Build history of the part. All positions in model axes, mm. A direction names the side the tool comes from. Round coordinates to 2 decimals unless told otherwise and drop trailing zeros. Write each loop counter-clockwise with the first axis right and the second up, starting at its lowest first coordinate (ties: lowest second). Pieces come first, ordered by that corner, then holes. Notation, with made-up numbers: (80, -33.5) - (93, -33.5) arc R29 ccw to (93, -9.5) - close; hole circle Ø9 at (-0.75, 2). An arc over 180 degrees is marked (long way). Answer as a JSON object with one key per item and string values. Group by question number.
Item 1: Probe line 1 (Y direction, x = 0, z = 4.5); line 2 (Z direction, x = -1, y = 3); line 3 (Y direction, x = -1, z = -4.25). List the from-to ranges inside material, lowest first. Write a range as from..to.
Item 2: Flat gauge pins, fed straight in: pin 1 (0.9 mm diameter, centred on y = 0.5, z = -5, fed in from +X); pin 2 (0.7 mm diameter, centred on y = 1.5, z = -1, fed in from -X). Where does each tip first touch, or does it go through?
Item 3: Which spindle directions (+Z, -Z, +X, -X, +Y, -Y) get a long thin tool onto all of the face, cutting with end or side? Do faces 1 (the flat face through (0, 3, 0)), 2 (the cylindrical face through (2.5, 0.1, 3.5)), 3 (the cylindrical face through (0, 2, -5)). Say none if no direction does.
Item 4: Slice it at A-A, the plane x = 0. List the corners of the cut face in (y, z).
Item 5: Slice it at B-B, the plane y = 0. List the corners of the cut face in (x, z), then the cut area to 3 significant figures.
Item 6: Two-plate mould, pull along Y, no slides. Class faces 4 (the cylindrical face through (3.34, 1.05, -0.1)), 5 (the flat face through (-1.5, 0, 1)), 6 (the flat face through (0, -3, 0)): +Y half, -Y half, draft (parallel to the pull), parting line (faces both ways), or undercut.
Item 7: Slice it at D-D, the plane x = 1. Give the number of separate pieces and of enclosed holes in the cut face, then the cut area to 3 significant figures.
Item 8: Slice it at C-C, the plane z = 5.75. List the corners of the cut face in (x, y).
from build123d import *
from build123d.topology import SkipClean

# Parameters (mm, degrees)
EXTRUDE_1_DEPTH                 = 7.5
EXTRUDE_1_DEPTH_BACK            = 7.5
SKETCH_1_R                      = 3.5
CUT_EXTRUDE_1_REACH             = 10.986
CUT_EXTRUDE_1_DIRECTION_2_REACH = 10.986
FILLET_1_R                      = 0.2
SKETCH_3_R                      = 2.5
CUT_EXTRUDE_2_DEPTH             = 0.5
CUT_EXTRUDE_3_DEPTH             = 7
CHAMFER_1_SIZE                  = 0.5
CHAMFER_2_SIZE                  = 0.5


with BuildPart() as part:
    # 草图1 → 凸台-拉伸1 (new, two sides: drawn at the far end of the back side and taken through both)
    with BuildSketch(Plane.XY.offset(-EXTRUDE_1_DEPTH_BACK)):
        Circle(SKETCH_1_R)
        with BuildLine():
            Line((-1.25, 1.5612495), (-1.25, -1.5612495))
            ThreePointArc((-1.25, -1.5612495), (0, -2), (1.25, -1.5612495))
            Line((1.25, -1.5612495), (1.25, 1.5612495))
            ThreePointArc((1.25, 1.5612495), (0, 2), (-1.25, 1.5612495))
        make_face(mode=Mode.SUBTRACT)
    extrude(amount=EXTRUDE_1_DEPTH + EXTRUDE_1_DEPTH_BACK)

    # 草图2 → 切除-拉伸1 (cut, up to next)
    with BuildSketch(Plane(origin=(0, 0, 0), x_dir=(1, 0, 0), z_dir=(0, 1, 0)), mode=Mode.PRIVATE) as cut_extrude_1_sk1:
        Polygon((0, 0), (-1.5, 0), (-1.5, 2.25), (1.5, 2.25), (1.5, 0), align=None)
    cut_extrude_1_tool1 = extrude(cut_extrude_1_sk1.sketch, amount=-CUT_EXTRUDE_1_REACH, mode=Mode.PRIVATE) & part.part
    add(cut_extrude_1_tool1.solids().sort_by_distance((0, 0, -1.125))[0], mode=Mode.SUBTRACT)

    # 草图2 → 切除-拉伸1 direction 2 (cut, up to next)
    with BuildSketch(Plane(origin=(0, 0, 0), x_dir=(1, 0, 0), z_dir=(0, 1, 0)), mode=Mode.PRIVATE) as cut_extrude_1_direction_2_sk1:
        Polygon((0, 0), (-1.5, 0), (-1.5, 2.25), (1.5, 2.25), (1.5, 0), align=None)
    cut_extrude_1_direction_2_tool1 = extrude(cut_extrude_1_direction_2_sk1.sketch, amount=CUT_EXTRUDE_1_DIRECTION_2_REACH, mode=Mode.PRIVATE) & part.part
    add(cut_extrude_1_direction_2_tool1.solids().sort_by_distance((0, 0, -1.125))[0], mode=Mode.SUBTRACT)

    # 圆角1
    fillet_1_edges = [part.edges().sort_by_distance(p)[0] for p in [
        (-3.5, 0, -7.5),
        (-3.5, 0, 7.5),
    ]]
    fillet(fillet_1_edges, radius=FILLET_1_R)

    # 草图3 → 切除-拉伸2 (cut)
    with BuildSketch(Plane.XY.offset(7.5)):
        Circle(SKETCH_3_R)
    extrude(amount=-CUT_EXTRUDE_2_DEPTH, mode=Mode.SUBTRACT)

    # 草图4 → 切除-拉伸3 (cut)
    with SkipClean():  # the faces are left unmerged after this step: merging them gives an invalid solid
        with BuildSketch(Plane.XY.offset(7)):
            with BuildLine():
                Line((-1.5, 0), (-1.5, 2))
                ThreePointArc((-1.5, 2), (2.5, 0), (-1.5, -2))
                Line((-1.5, -2), (-1.5, 0))
            make_face()
        extrude(amount=-CUT_EXTRUDE_3_DEPTH, mode=Mode.SUBTRACT)

    # 倒角1
    # the kernel refuses this chamfer: 0.5 mm, written as the material it takes off along each edge
    with BuildSketch(Plane(origin=(0, 0, 7.5), x_dir=(1, 0, 0), z_dir=(0, -1, 0))) as chamfer_1_piece_1_section:
        Polygon((2.5 + CHAMFER_1_SIZE, 0), (2.5, -CHAMFER_1_SIZE), (2.5, 0), align=None)
    chamfer_1_piece_1 = revolve(axis=Axis((0, 0, 7.5), (0, 0, 1)), mode=Mode.PRIVATE)
    chamfer_1_piece_1 = split(chamfer_1_piece_1, bisect_by=Plane(origin=(-1.5, 2.458621217, 7.265320049), z_dir=(1, 0, 0)), keep=Keep.TOP, mode=Mode.PRIVATE)
    chamfer_1_piece_1 = split(chamfer_1_piece_1, bisect_by=Plane(origin=(1.229310608, 2.458621217, 7), z_dir=(0, 0, 1)), keep=Keep.TOP, mode=Mode.PRIVATE)
    add(chamfer_1_piece_1, mode=Mode.SUBTRACT)
    with BuildSketch(Plane(origin=(0, 0, 7.5), x_dir=(1, 0, 0), z_dir=(0, -1, 0))) as chamfer_1_piece_2_section:
        Polygon((2.5 + CHAMFER_1_SIZE, 0), (2.5, -CHAMFER_1_SIZE), (2.5, 0), align=None)
    chamfer_1_piece_2 = revolve(axis=Axis((0, 0, 7.5), (0, 0, 1)), mode=Mode.PRIVATE)
    chamfer_1_piece_2 = split(chamfer_1_piece_2, bisect_by=Plane(origin=(-1.5, 0, 7.263385129), z_dir=(-1, 0, 0)), keep=Keep.TOP, mode=Mode.PRIVATE)
    chamfer_1_piece_2 = split(chamfer_1_piece_2, bisect_by=Plane(origin=(-2.750757007, 0, 7), z_dir=(0, 0, 1)), keep=Keep.TOP, mode=Mode.PRIVATE)
    add(chamfer_1_piece_2, mode=Mode.SUBTRACT)
    with BuildSketch(Plane(origin=(-1.5, -3.285841494, 7), x_dir=(0.02749587661058651, 0, -0.9996219169112968), z_dir=(0, 1, 0))) as chamfer_1_piece_3_section:
        Polygon((CHAMFER_1_SIZE * 0.999621916911, CHAMFER_1_SIZE * 0.0274958766106), (-CHAMFER_1_SIZE * 0.0274958766106, CHAMFER_1_SIZE * 0.999621916911), (0, 0), align=None)
    chamfer_1_piece_3 = extrude(amount=6.571682988, mode=Mode.PRIVATE)
    chamfer_1_piece_3 = chamfer_1_piece_3 & Plane(origin=(0, 0, 6.830829646), x_dir=(-0.5999999999999999, 0.8, 0), z_dir=(0, 0, 1)) * Cylinder(2.5, 16, mode=Mode.PRIVATE)
    add(chamfer_1_piece_3, mode=Mode.SUBTRACT)

    # 倒角2
    chamfer_2_edges = [part.edges().sort_by_distance(p)[0] for p in [
        (-1.25, 0, -7.5),
        (0, -2, -7.5),
        (1.25, 0, -7.5),
        (0, 2, -7.5),
    ]]
    chamfer(chamfer_2_edges, length=CHAMFER_2_SIZE)


solid = part.part
Geometry says:
{
 "1": {"line 1": "y = -3.5..-2.5, 2.5..3.5", "line 2": "z = -7.5..-2.25, 0..7.5", "line 3": "y = -3.35..-1.73, 1.73..3.35"},
 "2": {"pin 1": "stops at x = 3.5", "pin 2": "stops at x = -3.31"},
 "3": {"face 1": "+Y, -Y", "face 2": "+Z", "face 3": "+Z, -Z"},
 "4": {"outline": "(-3.5, -7.3) arc R0.2 ccw to (-3.3, -7.5) - (-2.5, -7.5) - (-2, -7) - (-2, -2.25) - (-3.5, -2.25) - close; (-3.5, 0) - (-2.5, 0) - (-2.5, 7) - (-3, 7.5) - (-3.3, 7.5) arc R0.2 ccw to (-3.5, 7.3) - close; (2, -7) - (2.5, -7.5) - (3.3, -7.5) arc R0.2 ccw to (3.5, -7.3) - (3.5, -2.25) - (2, -2.25) - close; (2.5, 0) - (3.5, 0) - (3.5, 7.3) arc R0.2 ccw to (3.3, 7.5) - (3, 7.5) - (2.5, 7) - close"},
 "5": {"outline": "(-3.5, -7.3) arc R0.2 ccw to (-3.3, -7.5) - (-1.75, -7.5) - (-1.25, -7) - (-1.25, -2.25) - (-1.5, -2.25) - (-1.5, 6.5) - (-2, 7) - (-2.5, 7) - (-3, 7.5) - (-3.3, 7.5) arc R0.2 ccw to (-3.5, 7.3) - close; (1.25, -7) - (1.75, -7.5) - (3.3, -7.5) arc R0.2 ccw to (3.5, -7.3) - (3.5, 7.3) arc R0.2 ccw to (3.3, 7.5) - (3, 7.5) - (2.5, 7) - (2.5, 0) - (1.5, 0) - (1.5, -2.25) - (1.25, -2.25) - close", "area": "54.0 mm^2"},
 "6": {"face 4": "parting line", "face 5": "undercut", "face 6": "draft"},
 "7": {"separate pieces": "4", "enclosed holes": "0", "area": "32.4 mm^2"},
 "8": {"outline": "circle Ø7 at (0, 0); hole (-1.5, -2) arc R2.5 ccw (long way) to (-1.5, 2) - close"}
}
